from build123d import *

# Parameters (mm, degrees)
SKETCH1_R                                   = 12.7
BOSS_EXTRUDE1_DEPTH                         = 3.5
CBORE_FOR_M3_CHEESE_HEAD_SCREW1_D           = 3.4
CBORE_FOR_M3_CHEESE_HEAD_SCREW1_CBORE_D     = 6.5
CBORE_FOR_M3_CHEESE_HEAD_SCREW1_CBORE_DEPTH = 2
SKETCH7_R                                   = 6.275
SKETCH7_R_2                                 = 4
BOSS_EXTRUDE2_DEPTH                         = 1
CHAMFER1_SIZE                               = 0.2


with BuildPart() as part:
    # Sketch1 → Boss-Extrude1 (new body)
    with BuildSketch(Plane.XY):
        Circle(SKETCH1_R)
    extrude(amount=BOSS_EXTRUDE1_DEPTH)

    # CBORE for M3 Cheese Head Screw1 (through all)
    with Locations(Plane(origin=(0, 0, 0), x_dir=(-1, 0, 0), z_dir=(0, 0, -1))):
        with Locations((4.694946795, -8.287526748), (-4.8297353, -8.209706568), (-9.524682095, 0.07782018), (-4.694946795, 8.287526748), (4.8297353, 8.209706568), (9.524682095, -0.07782018)):
            CounterBoreHole(CBORE_FOR_M3_CHEESE_HEAD_SCREW1_D / 2, CBORE_FOR_M3_CHEESE_HEAD_SCREW1_CBORE_D / 2, CBORE_FOR_M3_CHEESE_HEAD_SCREW1_CBORE_DEPTH)

    # Sketch7 → Boss-Extrude2 (add)
    with BuildSketch(Plane(origin=(0, 0, 0), x_dir=(-1, 0, 0), z_dir=(0, 0, -1))):
        Circle(SKETCH7_R)
        Circle(SKETCH7_R_2, mode=Mode.SUBTRACT)
    extrude(amount=BOSS_EXTRUDE2_DEPTH)

    # Chamfer1
    chamfer1_edges = [part.edges().sort_by_distance(p)[0] for p in [
        (4, 0, -1),
    ]]
    chamfer(chamfer1_edges, length=CHAMFER1_SIZE)


solid = part.part
Read the model definition and answer for the solid it produces. Units are mm, in the model's axes. A direction names the side the tool comes from. Round coordinates to 2 decimals unless told otherwise and drop trailing zeros. Write each loop counter-clockwise with the first axis right and the second up, starting at its lowest first coordinate (ties: lowest second). Pieces come first, ordered by that corner, then holes.
1. The part is cut by section D-D, the plane x = 0. Determine the outline of the cut face in (y, z) (3 decimals).
2. The part is cut by section C-C, the plane z = 2.65. Determine the outline of the cut face in (x, y).
3. Determine the mould class of faces 4 (the face through (-5.063, -9.947, 2.76)), 5 (the face through (8, -1, 2)), 6 (the face through (0, 0, 3.5)) for opening direction Z: pulls with the +Z half, pulls with the -Z half, needs draft (parallel to the pull), parting line crosses it, or undercut.
4. The part is cut by section B-B, the plane x = -4.5. Determine the outline of the cut face in (y, z), then the cut area to 3 significant figures.
5. The part is cut by section A-A, the plane y = -8.75. Determine the outline of the cut face in (x, z).
6. Which of the six approach directions +Z, -Z, +X, -X, +Y, -Y give full straight-line access (tool end or side, diameter ignored) to faces 1 (the face through (1.5, -4.1, -1)), 2 (the face through (0, 0, 0)), 3 (the face through (8, 5, 0))?
7. Straight lines are drawn through the part: L1, parallel to Y at x = 3.5, z = 0.05; L2, parallel to X at y = 6.5, z = 1.65; L3, parallel to Y at x = 3.75, z = 2.3. For each, find the intervals that lie inside material, in ascending order.
8. Given pin 1 Ø6 at (x, y) = (-2.5, -9) entering from -Z; pin 2 Ø8.5 at (x, y) = (-4.69, -8.29) entering from +Z; pin 3 Ø1.9 at (x, y) = (-3.5, 8) entering from -Z; pin 4 Ø1 at (x, z) = (4.5, 2) entering from +Y, each flat-ended and moving along its own axis, determine where each tip first touches the part or whether it passes through.
Values:
1. outline: (-12.7, 0) - (-6.275, 0) - (-6.275, -1) - (-4.2, -1) - (-4, -0.8) - (-4, 0) - (4, 0) - (4, -0.8) - (4.2, -1) - (6.275, -1) - (6.275, 0) - (12.7, 0) - (12.7, 3.5) - (-12.7, 3.5) - close
2. outline: circle Ø25.4 at (0, 0); hole circle Ø3.4 at (-9.52, -0.08); hole circle Ø3.4 at (-4.83, 8.21); hole circle Ø3.4 at (-4.69, -8.29); hole circle Ø3.4 at (4.69, 8.29); hole circle Ø3.4 at (4.83, -8.21); hole circle Ø3.4 at (9.52, 0.08)
3. face 4: needs draft
3. face 5: pulls with the -Z half
3. face 6: pulls with the +Z half
4. outline: (-11.88, 0) - (-11.53, 0) - (-11.53, 2) - (-9.98, 2) - (-9.98, 3.5) - (-11.88, 3.5) - close; (-6.6, 2) - (-5.04, 2) - (-5.04, 0) - (-4.37, 0) - (-4.37, -1) - (4.37, -1) - (4.37, 0) - (4.98, 0) - (4.98, 2) - (6.54, 2) - (6.54, 3.5) - (-6.6, 3.5) - close; (9.88, 2) - (11.44, 2) - (11.44, 0) - (11.88, 0) - (11.88, 3.5) - (9.88, 3.5) - close
4. area: 55.9 mm2
5. outline: (-9.2, 0) - (-7.91, 0) - (-7.91, 2) - (-6.33, 2) - (-6.33, 3.5) - (-9.2, 3.5) - close; (-3.06, 2) - (-1.48, 2) - (-1.48, 0) - (1.62, 0) - (1.62, 2) - (3.22, 2) - (3.22, 3.5) - (-3.06, 3.5) - close; (6.44, 2) - (8.03, 2) - (8.03, 0) - (9.2, 0) - (9.2, 3.5) - (6.44, 3.5) - close
6. face 1: -Z, +X, -X, +Y, -Y
6. face 2: -Z
6. face 3: -Z, +X, +Y
7. L1: y = -12.21 to -11.18, -5.24 to 5.27, 11.31 to 12.21
7. L2: x = -10.91 to -7.59, -2.07 to 1.98, 7.41 to 10.91
7. L3: y = -12.13 to -9.52, -6.9 to 6.87, 9.7 to 12.13
8. pin 1: stops at z = 0
8. pin 2: stops at z = 3.5
8. pin 3: stops at z = 2
8. pin 4: stops at y = 12.05
